Work out the finished part from the listing and answer in its coordinate system (mm). Give positions to 0.01 mm unless a question says otherwise; leave off trailing zeros. Loops run counter-clockwise (first coordinate to the right, second up) from the corner with the lowest first, then second, coordinate; pieces in that order, holes last. Notation, with made-up numbers: (52, -32.5) - (76, -32.5) arc R25 cw to (76, -2.5) - close; hole circle Ø1 at (65.5, 67). An arc over 180 degrees is marked (long way). One line per question, with ' | ' between items. Start each with the question number.
1. Section B-B (z = 0.75) is taken. Determine the outline of the cut face in (x, y) (3 decimals).
2. Find the intervals of material crossed by line 1 (X direction, y = -28, z = 1.35) (3 decimals); line 2 (X direction, y = 13, z = 1.9) (3 decimals); line 3 (Y direction, x = 27.5, z = 1.5) (3 decimals), in increasing order.
3. For a pull along Y with two mould halves and no side action, classify faces 1 (the face through (14.952, 11.138, 1.002)), 2 (the face through (33.11, -33.02, 1)), 3 (the face through (0, 0, 2.032)) as released by +Y, released by -Y, zero draft, split by the parting line, or undercut.
4. Section A-A (y = 12.7) is taken. Determine the outline of the cut face in (x, z) (3 decimals), plus the area to 3 significant figures.
5. This flat-tipped pin is pushed along its axis until it touches: pin 1 (10 mm diameter, centred on x = 26.5, y = -6.5, fed in from -Z). Where does it stop, or does it pass through?
Autodesk Inventor part; units mm, degrees
ref_plane "YZ Plane" through (0, 0, 0) normal (1, 0, 0) x (0, 1, 0)
ref_plane "XZ Plane" through (0, 0, 0) normal (0, 1, 0) x (-1, 0, 0)
ref_plane "XY Plane" through (0, 0, 0) normal (0, 0, 1) x (1, 0, 0)
sketch "Sketch1" plane through (0, 0, 0) normal (0, 0, 1) x (1, 0, 0)
  line L0 (28.575, -34.925) -> (-28.575, -34.925)
  line L1 (-34.925, -28.575) -> (-34.925, 28.575)
  line L2 (-28.575, 34.925) -> (28.575, 34.925)
  line L3 (34.925, 28.575) -> (34.925, -28.575)
  line L4 (34.925, -34.925) -> (-34.925, 34.925) construction
  line L5 (-34.925, -34.925) -> (34.925, 34.925) construction
  arc A0 (-28.575, 34.925) -> (-34.925, 28.575) centre (-28.575, 28.575) ccw
  arc A1 (34.925, 28.575) -> (28.575, 34.925) centre (28.575, 28.575) ccw
  arc A2 (28.575, -34.925) -> (34.925, -28.575) centre (28.575, -28.575) ccw
  arc A3 (-34.925, -28.575) -> (-28.575, -34.925) centre (-28.575, -28.575) ccw
  point P0 (0, 0)
  dimension "d0" = 69.85
  dimension "d1" = 69.85
  dimension "d2" = 6.35
extrude "Extrusion1" add sketch "Sketch1" along normal blind 2.032
sketch "Sketch2" plane through (0, 0, 2.032) normal (0, 0, 1) x (1, 0, 0)
  arc A0 (-28.575, 34.925) -> (-34.925, 28.575) centre (-28.575, 28.575) ccw
  arc A1 (34.925, 28.575) -> (28.575, 34.925) centre (28.575, 28.575) ccw
  arc A2 (28.575, -34.925) -> (34.925, -28.575) centre (28.575, -28.575) ccw
  arc A3 (-34.925, -28.575) -> (-28.575, -34.925) centre (-28.575, -28.575) ccw
  point P0 (0, 0)
hole "Hole1" at (-28.575, 28.575, 2.032) at (28.575, 28.575, 2.032) at (28.575, -28.575, 2.032) at (-28.575, -28.575, 2.032) direction (0, 0, -1) diameter 3.2 end through all
sketch "Sketch3" plane through (0, 0, 0) normal (0, 0, -1) x (-1, 0, 0)
  circle A0 centre (14.605, 12.7) radius 1.6
  circle A1 centre (-14.605, 12.7) radius 1.6
  line L0 (0, 49.4393) -> (0, -53.0853)
  point P0 (0, 0)
  dimension "d12" = 3.2
  dimension "d13" = 29.21
  dimension "d14" = 12.7
  dimension "d22" = 3.2
extrude "Extrusion2" cut sketch "Sketch3" against normal through all
equation "\"d0\" = d1"
equation "\"d22\" = d12"
properties part number "Durometer_Electronics_Enclosure-laser-cut"
Conclusion:
1) outline: (-34.925, -28.575) arc R6.35 ccw to (-28.575, -34.925) - (28.575, -34.925) arc R6.35 ccw to (34.925, -28.575) - (34.925, 28.575) arc R6.35 ccw to (28.575, 34.925) - (-28.575, 34.925) arc R6.35 ccw to (-34.925, 28.575) - close; hole circle Ø3.2 at (-28.575, -28.575); hole circle Ø3.2 at (-28.575, 28.575); hole circle Ø3.2 at (-14.605, 12.7); hole circle Ø3.2 at (14.605, 12.7); hole circle Ø3.2 at (28.575, -28.575); hole circle Ø3.2 at (28.575, 28.575)
2) line 1: -34.925 to -30.068, -27.082 to 27.082, 30.068 to 34.925 | line 2: -34.925 to -16.177, -13.033 to 13.033, 16.177 to 34.925 | line 3: -34.925 to -29.76, -27.39 to 27.39, 29.76 to 34.925
3) face 1: undercut | face 2: released by -Y | face 3: zero draft
4) outline: (-34.925, 0) - (-16.205, 0) - (-16.205, 2.032) - (-34.925, 2.032) - close; (-13.005, 0) - (13.005, 0) - (13.005, 2.032) - (-13.005, 2.032) - close; (16.205, 0) - (34.925, 0) - (34.925, 2.032) - (16.205, 2.032) - close | area: 129 mm²
5) pin 1: z = 0
